Read the model definition and answer for the solid it produces. Units are mm, in the model's axes. Round coordinates to 2 decimals unless told otherwise and drop trailing zeros. Order: outer loops, then holes, each group sorted by start corner. A loop starts at its lowest first (then second) coordinate and runs counter-clockwise, first axis right, second up. Notation, with made-up numbers: M 87,81.5 L 135,81.5 A13 cw 135,106.5 Z; hole C 81,-22 d9. An arc over 180 degrees is marked long. Use one line per item in the form item = value. Start each with the question number.
from build123d import *

# Parameters (mm, degrees)
F0_R     = 22.5
F1_DEPTH = 15
F3_D     = 8.2
F5_D     = 5.3
F6_R     = 2.25
F7_DEPTH = 50


with BuildPart() as f1:
    # F0 (on Top) → F1 (new body)
    with BuildSketch(Plane.XY):
        Circle(F0_R)
    extrude(amount=F1_DEPTH)

    # F3 (through all)
    with Locations(Plane.XY.offset(15)):
        with Locations((0, 0)):
            Hole(F3_D / 2)

    # F5 (through all)
    with Locations(Plane.XY.offset(15)):
        with Locations((0, 17), (14.722432, 8.5), (14.722432, -8.5), (0, -17), (-14.722432, -8.5), (-14.722432, 8.5)):
            Hole(F5_D / 2)

    # F6 (on Right) → F7 (cut, symmetric)
    with BuildSketch(Plane.YZ):
        with Locations((0, 11)):
            Circle(F6_R)
    extrude(amount=F7_DEPTH, both=True, mode=Mode.SUBTRACT)


solid = f1.part
Item 1: Find the intervals of material crossed by L1, parallel to Y at x = 0, z = 6.5; L2, parallel to X at y = -9, z = 3.25; L3, parallel to Y at x = 14.5, z = 13, in increasing order. Write a range as [from, to].
Item 2: Given P1, Ø3, axis at x = 12.5, z = 9, coming from the +Y side; P2, Ø6, axis at y = -12.5, z = 2.5, coming from the -X side; P3, Ø4, axis at y = -11, z = 2, coming from the -X side, each flat-ended and moving along its own axis, determine where each tip first touches the part or whether it passes through.
Item 3: Section D-D (y = -8.5) is taken. Write down the section's boundary in (x, z), and give its area (3 significant figures).
Item 4: For a pull along Y with two mould halves and no side action, classify faces 1 (the cylindrical face through (13.1, -0.29, 13.23)), 2 (the cylindrical face through (20.784, -8.618, 7.395)), 3 (the flat face through (5, 0, 15)) as pulls with the +Y half, pulls with the -Y half, needs draft (parallel to the pull), parting line crosses it, or undercut.
Item 5: Section B-B (y = 0) is taken. Write down the section's boundary in (x, z), and give its area (3 significant figures).
Item 6: Section C-C (x = -16) is taken. Write down the section's boundary in (y, z), and give its area (3 significant figures).
Item 7: Section A-A (x = 0) is taken. Write down the section's boundary in (y, z), and give its area (3 significant figures).
The answers:
q1.L1 = [-22.5, -19.65], [-14.35, -4.1], [4.1, 14.35], [19.65, 22.5]
q1.L2 = [-20.62, -17.32], [-12.12, 12.12], [17.32, 20.62]
q1.L3 = [-17.2, -11.14], [-5.86, -1.03], [1.03, 5.86], [11.14, 17.2]
q2.P1 = 19.63
q2.P2 = -20.4
q2.P3 = -20.62
q3.outline = M -20.83,0 L -17.37,0 L -17.37,15 L -20.83,15 Z; M -12.07,0 L 12.07,0 L 12.07,15 L -12.07,15 Z; M 17.37,0 L 20.83,0 L 20.83,15 L 17.37,15 Z
q3.area = 466 mm²
q4.face_1 = undercut
q4.face_2 = parting line crosses it
q4.face_3 = needs draft
q5.outline = M -22.5,0 L -4.1,0 L -4.1,8.75 L -22.5,8.75 Z; M -22.5,13.25 L -4.1,13.25 L -4.1,15 L -22.5,15 Z; M 4.1,0 L 22.5,0 L 22.5,8.75 L 4.1,8.75 Z; M 4.1,13.25 L 22.5,13.25 L 22.5,15 L 4.1,15 Z
q5.area = 386 mm²
q6.outline = M -15.82,0 L -10.82,0 L -10.82,15 L -15.82,15 Z; M -6.18,0 L 6.18,0 L 6.18,15 L -6.18,15 Z; M 10.82,0 L 15.82,0 L 15.82,15 L 10.82,15 Z; hole C 0,11 d4.5
q6.area = 319 mm²
q7.outline = M -22.5,0 L -19.65,0 L -19.65,15 L -22.5,15 Z; M -14.35,0 L -4.1,0 L -4.1,15 L -14.35,15 Z; M 4.1,0 L 14.35,0 L 14.35,15 L 4.1,15 Z; M 19.65,0 L 22.5,0 L 22.5,15 L 19.65,15 Z
q7.area = 393 mm²
